Autodesk Inventor part; units mm, degrees
ref_plane "YZ Plane" through (0, 0, 0) normal (1, 0, 0) x (0, 1, 0)
ref_plane "XZ Plane" through (0, 0, 0) normal (0, 1, 0) x (-1, 0, 0)
ref_plane "XY Plane" through (0, 0, 0) normal (0, 0, 1) x (1, 0, 0)
sketch "Sketch1" plane through (0, 0, 0) normal (0, 0, 1) x (1, 0, 0)
  line L0 (-16, 21) -> (16, 21)
  line L1 (21, 16) -> (21, -16)
  line L2 (16, -21) -> (-16, -21)
  line L3 (-21, -16) -> (-21, 16)
  circle A0 centre (-16, -16) radius 1.875
  circle A1 centre (-16, 16) radius 1.875
  circle A2 centre (16, 16) radius 1.875
  circle A3 centre (16, -16) radius 1.875
  circle A4 centre (0, 0) radius 20
  arc A5 (-16, 21) -> (-21, 16) centre (-16, 16) ccw
  arc A6 (21, 16) -> (16, 21) centre (16, 16) ccw
  arc A7 (16, -21) -> (21, -16) centre (16, -16) ccw
  arc A8 (-21, -16) -> (-16, -21) centre (-16, -16) ccw
  circle A9 centre (0, 0) radius 11
  circle A10 centre (0, 0) radius 9.8
  line L4 (-0.6, -10.9836) -> (-0.6, -19.991)
  line L5 (0.6, -10.9836) -> (0.6, -19.991)
  point P0 (21, -21)
  point P1 (21, 21)
  point P2 (-21, -21)
  dimension "d0" = 42
  dimension "d1" = 42
  dimension "d2" = 3.75
  dimension "d3" = 3.75
  dimension "d4" = 3.75
  dimension "d5" = 3.75
  dimension "d6" = 40
  dimension "d7" = 32
  dimension "d8" = 32
  dimension "d9" = 5
  dimension "d11" = 5
  dimension "d12" = 5
  dimension "d13" = 5
  dimension "d14" = 5
  dimension "d15" = 5
  dimension "d16" = 21
  dimension "d17" = 21
  dimension "d18" = 5
  dimension "d19" = 5
  dimension "d20" = 22
  dimension "d21" = 19.6
  dimension "d22" = 1.2
  dimension "d23" = 0.6
  dimension "d44" = 0
  dimension "d45" = 0
extrude "Base" add sketch "Sketch1" along normal blind 1.5 contours L0 A6 L1 A7 L2 A8 L3 A5 | A9
extrude "Support" add sketch "Sketch1" along normal blind 1.5 contours L4 A9 L5 A4 picked at (0.4667, -13.9909)
fillet "Fillet1" radius 2 4 edges at (-0.6, -10.9836, 0.75) (0.6, -10.9836, 0.75) (0.6, -19.991, 0.75) (-0.6, -19.991, 0.75)
pattern_circular "Support pattern" count 8 over 360 about axis through (0, 0, -10) along (0, 0, 1) of "Support", "Fillet1"
equation "\"d3\" = d2"
equation "\"d4\" = d2"
equation "\"d5\" = d2"
equation "\"d9\" = d13"
equation "\"d12\" = d11"
equation "\"d16\" = 0.5 * d0"
equation "\"d17\" = 0.5 * d0"
equation "\"d23\" = 0.5 * d22"
properties part number "40mm fan grill"
Build history of the part. All positions in model axes, mm. A direction names the side the tool comes from. Round coordinates to 2 decimals unless told otherwise and drop trailing zeros. Loops run counter-clockwise (first coordinate to the right, second up) from the corner with the lowest first, then second, coordinate; pieces in that order, holes last.
Item 1: Saw through at C-C (y = -13.5). List the corners of the cut face in (x, z), then the cut area to 3 significant figures.
Item 2: Pin check, flat tips, straight feed: P1, Ø3.5, axis at x = 16, y = -16, coming from the +Z side; P2, Ø12, axis at x = 13, y = -1, coming from the -Z side. Stop position of each tip, or through.
Item 3: Which spindle directions (+Z, -Z, +X, -X, +Y, -Y) get a long thin tool onto all of the face, cutting with end or side? Do faces 4 (the face through (-7.35, -8.853, 0.76)), 5 (the face through (19, 20, 1)). Say none if no direction does.
Item 4: Drill centre lines: line 1 along Y through (x, z) = (8, 1.1); line 2 along Y through (x, z) = (13, 1); line 3 along X through (y, z) = (15, 0.8). Where is each one in solid material? Low to high.
Item 5: Saw through at B-B (y = -3.5). List the corners of the cut face in (x, z).
Item 6: Two-plate mould, pull along Y, no slides. Class faces 1 (the face through (0, 21, 1)), 2 (the face through (20, -19, 1)), 3 (the face through (10.35, -11.2, 0.74)): released by +Y, released by -Y, zero draft, split by the parting line, or undercut.
Item 7: Saw through at A-A (x = 0). List the corners of the cut face in (y, z), then the cut area to 3 significant figures.
Worked answers:
1. outline: (-21, 0) - (-12.53, 0) - (-12.53, 1.5) - (-21, 1.5) - close; (-0.6, 0) - (0.6, 0) - (0.6, 1.5) - (-0.6, 1.5) - close; (12.53, 0) - (21, 0) - (21, 1.5) - (12.53, 1.5) - close
1. area: 27.2 mm2
2. P1: passes through
2. P2: stops at z = 0
3. face 4: +Z, -Z
3. face 5: +Z, -Z, +X, +Y
4. line 1: y = -21 to -18.33, -9.03 to -5.66, 5.66 to 9.03, 18.33 to 21
4. line 2: y = -21 to -12.15, -0.6 to 0.6, 12.15 to 21
4. line 3: x = -21 to -17.59, -14.41 to -12.67, -0.6 to 0.6, 12.67 to 14.41, 17.59 to 21
5. outline: (-21, 0) - (-19.69, 0) - (-19.69, 1.5) - (-21, 1.5) - close; (-10.43, 0) - (-9.15, 0) - (-9.15, 1.5) - (-10.43, 1.5) - close; (9.15, 0) - (10.43, 0) - (10.43, 1.5) - (9.15, 1.5) - close; (19.69, 0) - (21, 0) - (21, 1.5) - (19.69, 1.5) - close
6. face 1: released by +Y
6. face 2: released by -Y
6. face 3: undercut
7. outline: (-21, 0) - (-9.8, 0) - (-9.8, 1.5) - (-21, 1.5) - close; (9.8, 0) - (21, 0) - (21, 1.5) - (9.8, 1.5) - close
7. area: 33.6 mm2
